```python
from build123d import *

# Parameters (mm, degrees)
BOSS_EXTRUDE1_DEPTH = 3
SKETCH2_W           = 5
SKETCH2_H           = 15
CUT_EXTRUDE1_DEPTH  = 145.506055236
FILLET1_R           = 1


with BuildPart() as part:
    # Sketch1 → Boss-Extrude1 (new body)
    with BuildSketch(Plane(origin=(0, 0, 0), x_dir=(1, 0, 0), z_dir=(0, 1, 0))):
        Polygon((0, 67), (4, 67), (4, 47), (46, 47), (46, 28), (87, 28), (87, 47), (128, 47), (128, -7.5), (114, -7.5), (114, 0), (89, 0), (89, 14), (70, 14), (70, 0), (0, 0), align=None)
    extrude(amount=BOSS_EXTRUDE1_DEPTH)

    # Sketch2 → Cut-Extrude1 (cut, through all)
    with BuildSketch(Plane(origin=(0, 3, 0), x_dir=(1, 0, 0), z_dir=(0, 1, 0))):
        with Locations((115.5, 28.5)):
            Rectangle(SKETCH2_W, SKETCH2_H)
    extrude(amount=-CUT_EXTRUDE1_DEPTH, mode=Mode.SUBTRACT)

    # Fillet1
    fillet1_edges = [part.edges().sort_by_distance(p)[0] for p in [
        (4, 1.5, -47),
        (46, 1.5, -47),
        (46, 1.5, -28),
        (87, 1.5, -28),
        (87, 1.5, -47),
        (114, 1.5, 7.5),
        (114, 1.5, 0),
        (89, 1.5, 0),
        (89, 1.5, -14),
        (70, 1.5, -14),
        (70, 1.5, 0),
    ]]
    fillet(fillet1_edges, radius=FILLET1_R)


solid = part.part
```
Design review of the part built by this model. Coordinates are the model's own, in mm. A direction names the side the tool comes from. Round coordinates to 2 decimals unless told otherwise and drop trailing zeros. Write each loop counter-clockwise with the first axis right and the second up, starting at its lowest first coordinate (ties: lowest second). Pieces come first, ordered by that corner, then holes.
Item 1: The part is to be moulded in two halves that separate along X. For faces 5 (the flat face through (102, 1, 0)), 6 (the flat face through (0, 1, -33)), 7 (the flat face through (80, 1, -14)), 8 (the flat face through (115, 2, -21)), say which applies: +X half, -X half, draft (parallel to the pull), parting line (faces both ways), or undercut.
Item 2: For probe 1 along X at (y, z) = (1.7, -34); probe 2 along X at (y, z) = (1.05, -43.5); probe 3 along X at (y, z) = (0.6, -22.5), list the stretches that pass through material, from the lowest coordinate up.
Item 3: For faces 1 (the flat face through (46, 1, -38)), 2 (the flat face through (35, 1, 0)), 3 (the flat face through (89, 1, -7)), 4 (the flat face through (108, 1, -47)), list the 3-axis set-ups (+Z, -Z, +X, -X, +Y, -Y) from which the entire face can be reached by the end or side of a thin tool; tool diameter is ignored.
Item 4: Clearance check with flat-ended pins moving along their axes: pin 1 Ø1.5 at (x, y) = (106, 1.5) entering from +Z; pin 2 Ø0.9 at (y, z) = (2, -58.5) entering from +X; pin 3 Ø0.9 at (x, y) = (57, 2) entering from -Z. State where each tip first meets the part, or that it passes through.
Item 5: We need section D-D on x = 107. Write out the cut boundary in (y, z).
Item 6: We need section A-A on z = -34.5. Write out the cut boundary in (x, y), and give its area (3 significant figures).
Item 7: We need section B-B on z = -6. Write out the cut boundary in (x, y), and give its area (3 significant figures).
Returned:
1. face 5: draft
1. face 6: -X half
1. face 7: undercut
1. face 8: undercut
2. probe 1: x = 0 to 46, 87 to 113, 118 to 128
2. probe 2: x = 0 to 46, 87 to 128
2. probe 3: x = 0 to 113, 118 to 128
3. face 1: -Z, +Y, -Y
3. face 2: +Z, -X, +Y, -Y
3. face 3: +Z, +Y, -Y
3. face 4: -Z, +X, +Y, -Y
4. pin 1: stops at z = 0
4. pin 2: stops at x = 4
4. pin 3: stops at z = -28
5. outline: (0, -47) - (3, -47) - (3, 0) - (0, 0) - close
6. outline: (0, 0) - (46, 0) - (46, 3) - (0, 3) - close; (87, 0) - (113, 0) - (113, 3) - (87, 3) - close; (118, 0) - (128, 0) - (128, 3) - (118, 3) - close
6. area: 246 mm2
7. outline: (0, 0) - (70, 0) - (70, 3) - (0, 3) - close; (89, 0) - (128, 0) - (128, 3) - (89, 3) - close
7. area: 327 mm2
